Source: CAD feature listing. Evaluate the final solid. Frame: model axes, mm. Give positions to 0.01 mm unless a question says otherwise; leave off trailing zeros. Loops run counter-clockwise (first coordinate to the right, second up) from the corner with the lowest first, then second, coordinate; pieces in that order, holes last. Notation, with made-up numbers: (4, 62) - (13, 62) arc R18 ccw to (13, 87) - close; hole circle Ø8 at (46, 77). An arc over 180 degrees is marked (long way). Put each result on its own line as item: value.
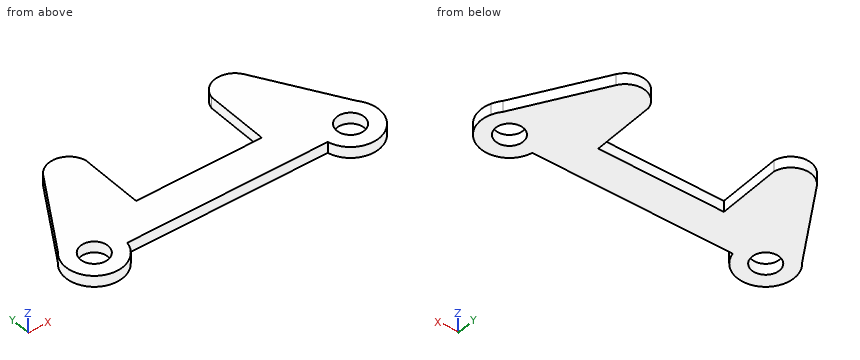
```python
from build123d import *

# Parameters (mm, degrees)
F0_R     = 2.475
F1_DEPTH = 2


with BuildPart() as f1:
    # F0 (on Top) → F1 (new body)
    with BuildSketch(Plane.XY):
        with BuildLine():
            ThreePointArc((-11.28048, 3.837689), (-14.25743, 6.713427), (-18.025508, 5.000625))
            Line((-18.025508, 5.000625), (-26.854825, -9.504681))
            ThreePointArc((-26.854825, -9.504681), (-25.355263, -17.480133), (-17.990624, -14.071526))
            Line((-17.990624, -14.071526), (0, -14.071526))
            Line((0, -14.071526), (17.990624, -14.071526))
            ThreePointArc((17.990624, -14.071526), (24.515641, -17.822764), (27.794171, -11.047893))
            Line((27.794171, -11.047893), (26.854825, -9.504681))
            Line((26.854825, -9.504681), (18.025508, 5.000625))
            ThreePointArc((18.025508, 5.000625), (14.25743, 6.713427), (11.28048, 3.837689))
            Line((11.28048, 3.837689), (11.28048, -7.571526))
            Line((11.28048, -7.571526), (0, -7.571526))
            Line((0, -7.571526), (-11.28048, -7.571526))
            Line((-11.28048, -7.571526), (-11.28048, 3.837689))
        make_face()
        with Locations((-23, -12.90859)):
            Circle(F0_R, mode=Mode.SUBTRACT)
        with Locations((23, -12.90859)):
            Circle(F0_R, mode=Mode.SUBTRACT)
        with BuildLine():
            Line((26.854825, -9.504681), (27.794171, -11.047893))
            ThreePointArc((27.794171, -11.047893), (27.392796, -10.234714), (26.854825, -9.504681))
        make_face()
    extrude(amount=F1_DEPTH)


solid = f1.part
```
1) Section query C-C, the plane z = 1. State how many separate pieces and enclosed holes the cut face has, plus the area to 3 significant figures.
Check result:
separate pieces: 1
enclosed holes: 2
area: 658 mm²
2) Section query D-D, the plane x = 5. Output: boundary loops of the cut face in (y, z).
Check result:
outline: (-14.07, 0) - (-7.57, 0) - (-7.57, 2) - (-14.07, 2) - close
3) Section query B-B, the plane y = 4.5. Output: boundary loops of the cut face in (x, z).
Check result:
outline: (-18.33, 0) - (-11.49, 0) - (-11.49, 2) - (-18.33, 2) - close; (11.49, 0) - (18.33, 0) - (18.33, 2) - (11.49, 2) - close
4) Section query A-A, the plane x = 23. Output: boundary loops of the cut face in (y, z).
Check result:
outline: (-18.05, 0) - (-15.38, 0) - (-15.38, 2) - (-18.05, 2) - close; (-10.43, 0) - (-3.17, 0) - (-3.17, 2) - (-10.43, 2) - close
5) Pin query (flat end, axial travel): P1, Ø1, axis at x = -5.5, z = 0.5, coming from the +Y side; P2, Ø1, axis at y = -0.5, z = 0, coming from the +X side; P3, Ø3, axis at x = 23, y = -12.91, coming from the -Z side; P4, Ø1, axis at y = -1.5, z = 1, coming from the +X side. Return the tip coordinate at first contact, or that it passes through.
Check result:
P1: y = -7.57
P2: x = 21.68
P3: through
P4: x = 22.29
6) Material intervals for line 1 along X through (y, z) = (-12.75, 0.85); line 2 along X through (y, z) = (-15, 0.3); line 3 along X through (y, z) = (-14, 0.5), sorted ascending. Write a range as [from, to].
Check result:
line 1: [-28.14, -25.47], [-20.53, 20.53], [25.47, 28.14]
line 2: [-27.7, -24.32], [-21.68, -18.3], [18.3, 21.68], [24.32, 27.7]
line 3: [-28.03, -25.22], [-20.78, 20.78], [25.22, 28.03]
